Read the model definition and answer for the solid it produces. Units are mm, in the model's axes. Coordinates: 2 decimals unless noted, no trailing zeros. Order: outer loops, then holes, each group sorted by start corner. A loop starts at its lowest first (then second) coordinate and runs counter-clockwise, first axis right, second up.
```python
from build123d import *

# Parameters (mm, degrees)
F0_W     = 400
F0_H     = 350
F1_DEPTH = 19
F3_DEPTH = 19.001
F5_DEPTH = 19.001
F6_R     = 24.466171
F7_DEPTH = 19.001


with BuildPart() as f1:
    # F0 (on Top) → F1 (new body)
    with BuildSketch(Plane.XY):
        Rectangle(F0_W, F0_H)
    extrude(amount=F1_DEPTH)

    # F2 (on face) → F3 (cut, through all)
    with BuildSketch(Plane.XY.offset(19)):
        with BuildLine():
            ThreePointArc((-200, 129.103959), (-177.466349, 162.178838), (-139.554203, 175))
            Line((-139.554203, 175), (-200, 175))
            Line((-200, 175), (-200, 129.103959))
        make_face()
    extrude(amount=-F3_DEPTH, mode=Mode.SUBTRACT)

    # F4 (on face) → F5 (cut, through all)
    with BuildSketch(Plane.XY.offset(19)):
        with BuildLine():
            ThreePointArc((200, -128.668547), (179.591152, -157.638715), (148.698151, -175))
            Line((148.698151, -175), (200, -175))
            Line((200, -175), (200, -128.668547))
        make_face()
    extrude(amount=-F5_DEPTH, mode=Mode.SUBTRACT)

    # F6 (on face) → F7 (cut, through all)
    with BuildSketch(Plane(origin=(0, 0, 0), x_dir=(1, 0, 0), z_dir=(0, 0, -1))):
        with Locations((162.81534, -136.567061)):
            Circle(F6_R)
    extrude(amount=-F7_DEPTH, mode=Mode.SUBTRACT)


solid = f1.part
```
1) Determine the mould class of faces 1 (the cylindrical face through (143.4, 151.454, 9.367)), 2 (the cylindrical face through (-177.92, 161.83, 9.63)), 3 (the flat face through (-28, -175, 9)) for opening direction X: pulls with the +X half, pulls with the -X half, needs draft (parallel to the pull), parting line crosses it, or undercut.
A:
face 1: undercut
face 2: pulls with the -X half
face 3: needs draft
2) A cutting plane is placed at A-A, the plane z = 15.5. Determine the outline of the cut face in (x, y).
A:
outline: (-200, -175) - (148.7, -175) arc R80.28 ccw to (200, -128.67) - (200, 175) - (-139.55, 175) arc R62.98 ccw to (-200, 129.1) - close; hole circle Ø48.93 at (162.82, 136.57)
3) Straight lines are drawn through the part: line 1 (X direction, y = 131, z = 5); line 2 (Y direction, x = 179, z = 8); line 3 (X direction, y = 134, z = 17.5). For each, find the intervals that lie inside material, in ascending order.
A:
line 1: x = -199.43 to 138.99, 186.64 to 200
line 2: y = -158.17 to 118.22, 154.92 to 175
line 3: x = -198.4 to 138.48, 187.15 to 200
4) A flat-ended cylindrical pin translates along its axis: pin 1 Ø8 at (x, y) = (-150.5, -64) entering from -Z. Find the tip coordinate at first contact, or state that the pin passes through.
A:
pin 1: stops at z = 0
